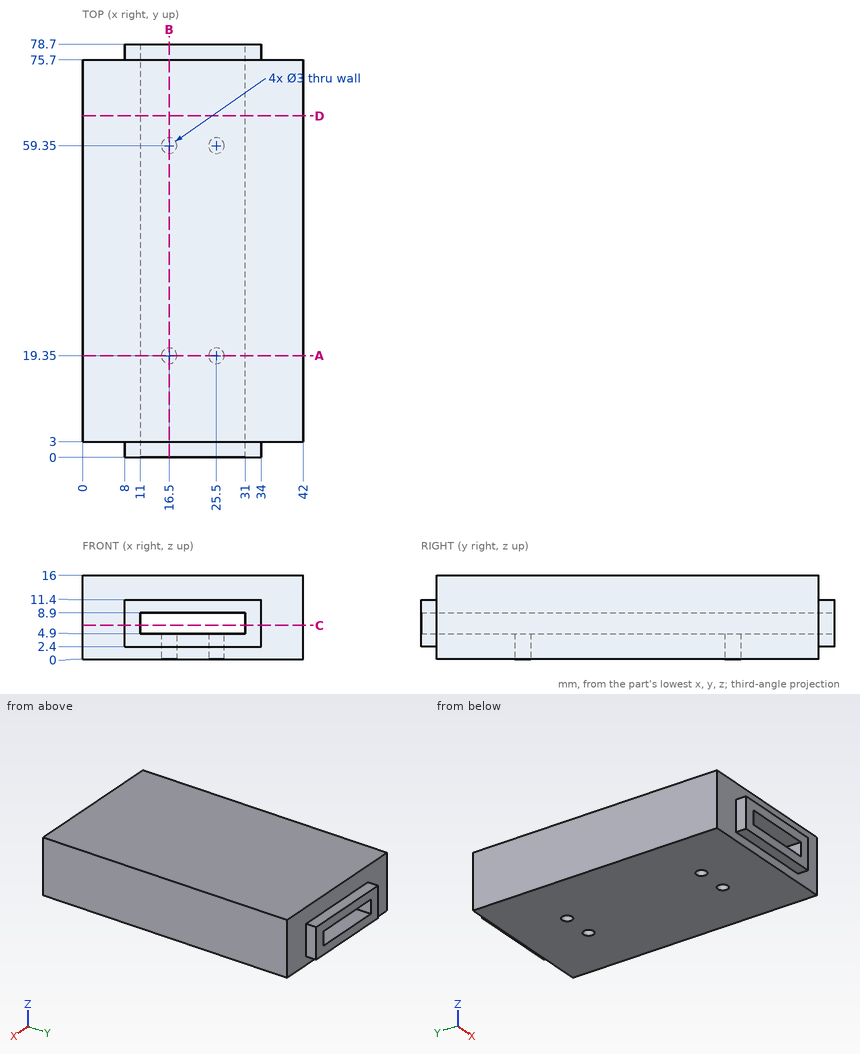
Geometry: see drawing. Coordinates: mm, zero at the bounding-box minimum. Round coordinates to 2 decimals unless told otherwise and drop trailing zeros. Loops run counter-clockwise (first coordinate to the right, second up) from the corner with the lowest first, then second, coordinate; pieces in that order, holes last. Notation, with made-up numbers: (-22, 27.25) -> (36, 27.25) arc R12 ccw to (36, 46.25) -> close; hole circle Ø10 at (70, -5.5). An arc over 180 degrees is marked (long way). Use one line per item in the form item = value. Start each with the question number.
Item 1: Section query D-D on y = 65. Return the cut outline in (x, z).
Item 2: Contact query for flat-ended pins moving along their axis: pin 1 Ø1.5 at (x, y) = (22, 1.5) entering from -Z; pin 2 Ø1.5 at (y, z) = (1.5, 8.5) entering from +X; pin 3 Ø1.5 at (y, z) = (77.5, 5) entering from -X. Output: stop coordinate, or through.
Item 3: Material intervals for L1, parallel to Y at x = 25.5, z = 2.2; L2, parallel to Y at x = 16.5, z = 3.65; L3, parallel to X at y = 19.35, z = 3.3, sorted ascending. Write a range as from..to.
Item 4: Section query C-C on z = 6.5. Return the cut outline in (x, y), then the cut area to 3 significant figures.
Item 5: Section query B-B on x = 16.5. Return the cut outline in (y, z).
Item 6: Section query A-A on y = 19.35. Return the cut outline in (x, z).
Ans:
q1.outline = (0, 0) -> (42, 0) -> (42, 16) -> (0, 16) -> close; hole (11, 4.9) -> (31, 4.9) -> (31, 8.9) -> (11, 8.9) -> close
q2.pin_1 = 2.4
q2.pin_2 = 34
q2.pin_3 = 8
q3.L1 = 3..17.85, 20.85..57.85, 60.85..75.7
q3.L2 = 0..17.85, 20.85..57.85, 60.85..78.7
q3.L3 = 0..15, 18..24, 27..42
q4.outline = (0, 3) -> (8, 3) -> (8, 0) -> (11, 0) -> (11, 78.7) -> (8, 78.7) -> (8, 75.7) -> (0, 75.7) -> close; (31, 0) -> (34, 0) -> (34, 3) -> (42, 3) -> (42, 75.7) -> (34, 75.7) -> (34, 78.7) -> (31, 78.7) -> close
q4.area = 1,640 mm^2
q5.outline = (0, 2.4) -> (3, 2.4) -> (3, 0) -> (17.85, 0) -> (17.85, 4.9) -> (0, 4.9) -> close; (0, 8.9) -> (78.7, 8.9) -> (78.7, 11.4) -> (75.7, 11.4) -> (75.7, 16) -> (3, 16) -> (3, 11.4) -> (0, 11.4) -> close; (20.85, 0) -> (57.85, 0) -> (57.85, 4.9) -> (20.85, 4.9) -> close; (60.85, 0) -> (75.7, 0) -> (75.7, 2.4) -> (78.7, 2.4) -> (78.7, 4.9) -> (60.85, 4.9) -> close
q6.outline = (0, 0) -> (15, 0) -> (15, 4.9) -> (11, 4.9) -> (11, 8.9) -> (31, 8.9) -> (31, 4.9) -> (27, 4.9) -> (27, 0) -> (42, 0) -> (42, 16) -> (0, 16) -> close; (18, 0) -> (24, 0) -> (24, 4.9) -> (18, 4.9) -> close
